from build123d import *

# Parameters (mm, degrees)
F1_DEPTH = 20
F2_W     = 140
F2_H     = 34
F3_DEPTH = 60
F4_R     = 6
F5_DEPTH = 50


with BuildPart() as f1:
    # F0 (on Front) → F1 (new body, symmetric)
    with BuildSketch(Plane.XZ):
        with BuildLine():
            Line((40, 25), (-60, 25))
            Line((-60, 25), (-60, -25))
            Line((-60, -25), (40, -25))
            ThreePointArc((40, -25), (54.142136, -19.142136), (60, -5))
            Line((60, -5), (60, 5))
            ThreePointArc((60, 5), (54.142136, 19.142136), (40, 25))
        make_face()
    extrude(amount=F1_DEPTH, both=True)

    # F2 (on face) → F3 (cut)
    with BuildSketch(Plane.XY.offset(25)):
        with Locations((13, 0)):
            Rectangle(F2_W, F2_H)
    extrude(amount=-F3_DEPTH, mode=Mode.SUBTRACT)

    # F4 (on face) → F5 (cut)
    with BuildSketch(Plane(origin=(0, 20, 0), x_dir=(-1, 0, 0), z_dir=(0, 1, 0))):
        with Locations((3.8, 0)):
            Circle(F4_R)
    extrude(amount=-F5_DEPTH, mode=Mode.SUBTRACT)


solid = f1.part
CAD build for the part. Positions are in the model's coordinates, mm. A direction names the side the tool comes from. Give positions to 0.01 mm unless a question says otherwise; leave off trailing zeros. Write each loop counter-clockwise with the first axis right and the second up, starting at its lowest first coordinate (ties: lowest second). Pieces come first, ordered by that corner, then holes. Notation, with made-up numbers: (-33.5, -5.75) - (18.5, -5.75) arc R18 ccw to (18.5, 16.25) - close; hole circle Ø7 at (35.25, 12). An arc over 180 degrees is marked (long way). Answer as CSV lines item,"result".
Q1. Pull direction X, two halves, no side cores. Call faces 1 (the face through (-57, 0, 0)), 2 (the face through (-1, 20, 6)), 3 (the face through (2.194, -18.479, 0.264)): released by +X, released by -X, zero draft, split by the parting line, or undercut.
Result set:
face 1,"released by +X"
face 2,"zero draft"
face 3,"undercut"
Q2. Band-saw the part on D-D (y = -10). Give the cut face in (x, z), and give its area (3 significant figures).
Result set:
outline,"(-60, -25) - (-57, -25) - (-57, 25) - (-60, 25) - close"
area,"150 mm²"
Q3. Band-saw the part on C-C (x = -38). Give the cut face in (y, z).
Result set:
outline,"(-20, -25) - (-17, -25) - (-17, 25) - (-20, 25) - close; (17, -25) - (20, -25) - (20, 25) - (17, 25) - close"
Q4. Band-saw the part on A-A (x = -3.8). Give the cut face in (y, z).
Result set:
outline,"(-20, -25) - (-17, -25) - (-17, -6) - (-20, -6) - close; (-20, 6) - (-17, 6) - (-17, 25) - (-20, 25) - close; (17, -25) - (20, -25) - (20, -6) - (17, -6) - close; (17, 6) - (20, 6) - (20, 25) - (17, 25) - close"
Q5. 3-axis set-ups, long thin cutter, end or side, ignore diameter. For faces 4 (the face through (53.986, 18.479, -19.297)), 5 (the face through (1, -17, 6)): which of +Z, -Z, +X, -X, +Y, -Y reach the whole face in a straight line?
Result set:
face 4,"-Z, +X, +Y, -Y"
face 5,"+Z, -Z, +X"
Q6. Flat gauge pins, fed straight in: pin 1 Ø11 at (x, z) = (-3.8, 0) entering from -Y; pin 2 Ø1 at (y, z) = (7, 0) entering from +X. Where does each tip first touch, or does it go through?
Result set:
pin 1,"through"
pin 2,"x = -57"
Q7. Drill centre lines: line 1 (Y direction, x = -15.5, z = 19.5); line 2 (Z direction, x = -3.8, y = 18.5); line 3 (Z direction, x = -3, y = -18). Where is each one in solid material? Low to high. Write a range as from..to.
Result set:
line 1,"-20..-17, 17..20"
line 2,"-25..-6, 6..25"
line 3,"-25..-5.95, 5.95..25"
Q8. Band-saw the part on B-B (z = 0). Give the cut face in (x, y), and give its area (3 significant figures).
Result set:
outline,"(-60, -20) - (-9.8, -20) - (-9.8, -17) - (-57, -17) - (-57, 17) - (-9.8, 17) - (-9.8, 20) - (-60, 20) - close; (2.2, -20) - (60, -20) - (60, -17) - (2.2, -17) - close; (2.2, 17) - (60, 17) - (60, 20) - (2.2, 20) - close"
area,"750 mm²"
